Geometry: final body of the model. Coordinates: model frame, mm. Face numbers are marked on the shaded views. A direction names the side the tool comes from. Give positions to 0.01 mm unless a question says otherwise; leave off trailing zeros. Loops run counter-clockwise (first coordinate to the right, second up) from the corner with the lowest first, then second, coordinate; pieces in that order, holes last.
1. Material intervals for line 1 along Y through (x, z) = (1.25, 2.5); line 2 along X through (y, z) = (30.5, 0.25); line 3 along X through (y, z) = (35.5, -3.25), sorted ascending.
2. Section B-B, the plane x = 0. Output: boundary loops of the cut face in (y, z) (3 decimals).
3. First-contact query: P1, Ø4, axis at x = 3, y = 8, coming from the -Z side; P2, Ø3, axis at x = -0.5, z = -2, coming from the +Y side; P3, Ø2, axis at y = 15.5, z = -3.5, coming from the +X side; P4, Ø1, axis at x = 3.5, z = -2.5, coming from the +Y side. Flat tips, straight axial feed; report the tip coordinate or a pass-through.
4. Section A-A, the plane z = 0. Output: boundary loops of the cut face in (x, y) (3 decimals).
5. Access query for the marked faces 1 and 2. Directions: +Z, -Z, +X, -X, +Y, -Y. A direction counts if a zero-diameter tool reaches every point of the face in a straight line with its end or side. Return the directions, or none.
6. Section C-C, the plane y = 21.5. Output: boundary loops of the cut face in (x, z), then the cut area to 3 significant figures.
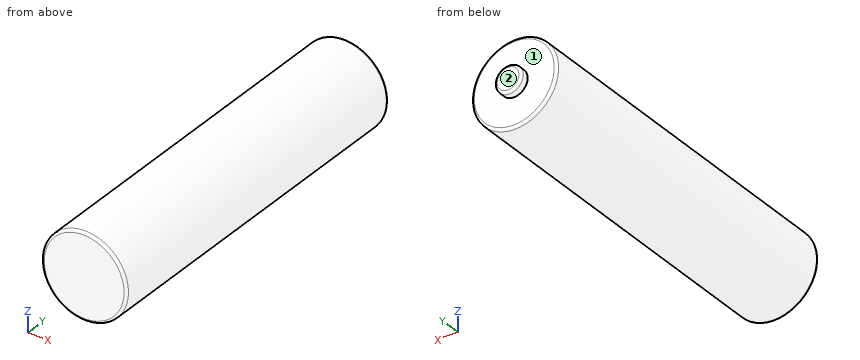
from build123d import *

# Parameters (mm, degrees)
SKETCH1_R           = 5
BOSS_EXTRUDE1_DEPTH = 42
SKETCH2_R           = 1.575
BOSS_EXTRUDE2_DEPTH = 1
FILLET1_R           = 0.3


with BuildPart() as part:
    # Sketch1 → Boss-Extrude1 (new body)
    with BuildSketch(Plane(origin=(0, 0, 0), x_dir=(1, 0, 0), z_dir=(0, 1, 0))):
        Circle(SKETCH1_R)
    extrude(amount=BOSS_EXTRUDE1_DEPTH)

    # Sketch2 → Boss-Extrude2 (add)
    with BuildSketch(Plane(origin=(0, 42, 0), x_dir=(1, 0, 0), z_dir=(0, 1, 0))):
        Circle(SKETCH2_R)
    extrude(amount=BOSS_EXTRUDE2_DEPTH)

    # Fillet1
    fillet1_edges = [part.edges().sort_by_distance(p)[0] for p in [
        (-5, 0, 0),
        (-5, 42, 0),
        (-1.575, 43, 0),
    ]]
    fillet(fillet1_edges, radius=FILLET1_R)


solid = part.part
Answers below:
1. line 1: y = 0 to 42
1. line 2: x = -4.99 to 4.99
1. line 3: x = -3.8 to 3.8
2. outline: (0, -4.7) arc R0.3 ccw to (0.3, -5) - (41.7, -5) arc R0.3 ccw to (42, -4.7) - (42, -1.575) - (42.7, -1.575) arc R0.3 ccw to (43, -1.275) - (43, 1.275) arc R0.3 ccw to (42.7, 1.575) - (42, 1.575) - (42, 4.7) arc R0.3 ccw to (41.7, 5) - (0.3, 5) arc R0.3 ccw to (0, 4.7) - close
3. P1: stops at z = -4.9
3. P2: stops at y = 43
3. P3: stops at x = 4.33
3. P4: stops at y = 42
4. outline: (-5, 0.3) arc R0.3 ccw to (-4.7, 0) - (4.7, 0) arc R0.3 ccw to (5, 0.3) - (5, 41.7) arc R0.3 ccw to (4.7, 42) - (1.575, 42) - (1.575, 42.7) arc R0.3 ccw to (1.275, 43) - (-1.275, 43) arc R0.3 ccw to (-1.575, 42.7) - (-1.575, 42) - (-4.7, 42) arc R0.3 ccw to (-5, 41.7) - close
5. face 1: +Y
5. face 2: +Z, -Z, +X, -X, +Y
6. outline: circle Ø10 at (0, 0)
6. area: 78.5 mm2
